from build123d import *

# Parameters (mm, degrees)
SKETCH067_R             = 1.875
PAD035_DEPTH            = 4.75
SKETCH068_R             = 3
POCKET007018_DEPTH      = 3.75
POCKET007019_DEPTH      = 3.5
FILLET001_R             = 3
BODY008_PLACEMENT_ANGLE = 180


with BuildPart() as part:
    # Sketch067 → Pad035 (new body)
    with BuildSketch(Plane.XY.offset(-4)):
        with BuildLine():
            Line((17, -30.839247), (30.583921, -30.839247))
            Line((30.583921, -30.839247), (30.583921, -40.999999))
            ThreePointArc((30.583921, -40.999999), (36.500001, -45.999999), (42.416081, -40.999999))
            Line((42.416081, -30.839247), (42.416081, -40.999999))
            Line((42.416081, -30.839247), (55.233103, -30.839247))
            Line((55.233103, -30.839247), (83.336753, 5.788599))
            Line((83.336753, 5.788599), (75.403023, 11.875956))
            Line((75.403023, 11.875956), (48.766897, -22.839247))
            Line((48.766897, -22.839247), (17, -22.839247))
            Line((17, -22.839247), (17, -30.839247))
        make_face()
        with Locations((21, -26.839247)):
            Circle(SKETCH067_R, mode=Mode.SUBTRACT)
        with Locations((52, -26.839247)):
            Circle(SKETCH067_R, mode=Mode.SUBTRACT)
        with BuildLine():
            ThreePointArc((38.875001, -34.999999), (36.500001, -32.624999), (34.125001, -34.999999))
            Line((34.125001, -34.999999), (34.125001, -40.999999))
            ThreePointArc((34.125001, -40.999999), (36.500001, -43.374999), (38.875001, -40.999999))
            Line((38.875001, -34.999999), (38.875001, -40.999999))
        make_face(mode=Mode.SUBTRACT)
        with BuildLine():
            ThreePointArc((77.601735, 2.626292), (77.163221, 5.9563), (73.833213, 5.517786))
            Line((73.833213, 5.517786), (70.789534, 1.550921))
            ThreePointArc((70.789534, 1.550921), (71.228048, -1.779087), (74.558056, -1.340574))
            Line((77.601735, 2.626292), (74.558056, -1.340574))
        make_face(mode=Mode.SUBTRACT)
    extrude(amount=PAD035_DEPTH)

    # Sketch068 (on ShapeBinder) → Pocket007018 (cut)
    with BuildSketch(Plane(origin=(-1.5, -35, 0.75), x_dir=(0, 1, 0), z_dir=(0, 0, -1))):
        with Locations((8.353044, 53.594845)):
            Circle(SKETCH068_R)
        with Locations((8.160753, 22.5)):
            Circle(SKETCH068_R)
    extrude(amount=POCKET007018_DEPTH, mode=Mode.SUBTRACT)

    # Sketch069 → Pocket007019 (cut)
    with BuildSketch(Plane.XY.offset(-4)):
        Polygon((40.125001, -37.092894), (40.125001, -32.907104), (36.500001, -30.814209), (32.875001, -32.907104), (32.875001, -37.092894), (32.875001, -38.907104), (32.875001, -43.092894), (36.500001, -45.185788), (40.125001, -43.092894), (40.125001, -38.907104), align=None)
        Polygon((77.319431, 0.204926), (79.867471, 3.525818), (78.265513, 7.392932), (74.115516, 7.939152), (71.567477, 4.61826), (71.071837, 3.972287), (68.523798, 0.651395), (70.125755, -3.215719), (74.275752, -3.76194), (76.823792, -0.441047), align=None)
    extrude(amount=POCKET007019_DEPTH, mode=Mode.SUBTRACT)

    # Fillet001
    fillet001_edges = [part.edges().sort_by_distance(p)[0] for p in [
        (42.416081, -30.839247, -1.625),
        (55.233103, -30.839247, -1.625),
        (83.336753, 5.788599, -1.625),
        (75.403023, 11.875956, -1.625),
        (48.766897, -22.839247, -1.625),
        (17, -22.839247, -1.625),
        (17, -30.839247, -1.625),
        (30.583921, -30.839247, -1.625),
    ]]
    fillet(fillet001_edges, radius=FILLET001_R)


with BuildPart() as part_1:
    # Body008 placement: moved
    add(part.part.rotate(Axis((0, 0, 0), (1, 0, 0)), BODY008_PLACEMENT_ANGLE))


solid = part_1.part
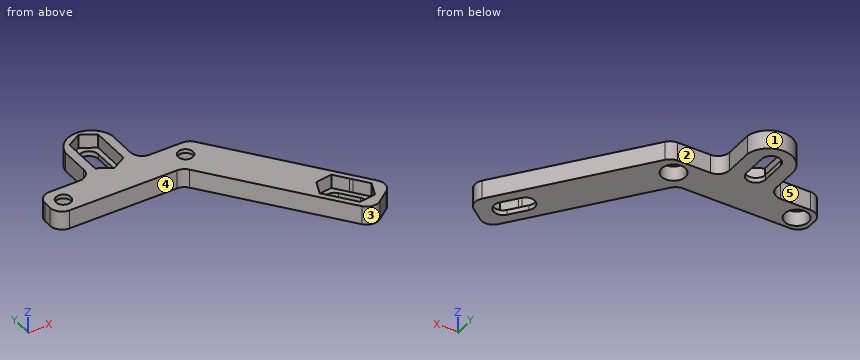
For this review, take the finished solid that the model builds, in its own axes (mm). Face numbers are marked on the shaded views. A direction names the side the tool comes from. Round coordinates to 2 decimals unless told otherwise and drop trailing zeros. Loops run counter-clockwise (first coordinate to the right, second up) from the corner with the lowest first, then second, coordinate; pieces in that order, holes last. Notation, with made-up numbers: (-11.75, 64.25) - (17.25, 64.25) arc R29 cw to (17.25, 87.25) - close; hole circle Ø6 at (11.25, 78). An arc over 180 degrees is marked (long way). Put each result on its own line as item: value. Start each with the question number.
1. Consider section C-C on z = 1.45. State how many separate pieces and enclosed holes the cut face has, plus the area to 3 significant figures.
2. For the marked faces 1, 2, 3, 4 and 5, list the 3-axis set-ups (+Z, -Z, +X, -X, +Y, -Y) from which the entire face can be reached by the end or side of a thin tool; tool diameter is ignored.
3. Consider section A-A on x = 21. State the section outline as (y, z) points.
4. For probe 1 along X at (y, z) = (38, 3.2) (3 decimals); probe 2 along Y at (x, z) = (21, 3.75); probe 3 along Y at (x, z) = (50.5, 1.85), list the stretches that pass through material, from the lowest coordinate up. Write a range as [from, to].
5. Insertion check: P1, Ø9, axis at x = 74, y = -4.5, coming from the +Z side; P2, Ø2, axis at x = 62.5, z = 2, coming from the +Y side; P3, Ø1.4, axis at y = 39, z = 2.5, coming from the -X side; P4, Ø1.8, axis at x = 53, y = 28, coming from the -Z side. Each pin has a flat end and moves straight along its axis. Give the tip position at first contact, or say it passes through.
6. Consider section B-B on x = 67. State the section outline as (y, z) points.
7. Consider section D-D on x = 48. State the section outline as (y, z) points, plus the area to 3 significant figures.
Result sheet:
1. separate pieces: 1
1. enclosed holes: 4
1. area: 663 mm^2
2. face 1: +Z, -Z, +Y
2. face 2: +Z, -Z, +X, +Y
2. face 3: +Z, -Z, -Y
2. face 4: +Z, -Z, -X, -Y
2. face 5: +Z, -Z, -X, +Y
3. outline: (22.84, -0.75) - (23.84, -0.75) - (23.84, 3) - (24.96, 3) - (24.96, 4) - (22.84, 4) - close; (28.71, 3) - (29.84, 3) - (29.84, -0.75) - (30.84, -0.75) - (30.84, 4) - (28.71, 4) - close
4. probe 1: [30.584, 32.875], [40.125, 42.416]
4. probe 2: [22.84, 24.96], [28.71, 30.84]
4. probe 3: [20.58, 24.11], [29.19, 30.84]
5. P1: z = 4
5. P2: y = 22.67
5. P3: x = 30.58
5. P4: z = 3
6. outline: (-0.92, -0.75) - (15.5, -0.75) - (15.5, 4) - (-0.92, 4) - close
7. outline: (22.75, -0.75) - (30.84, -0.75) - (30.84, 4) - (22.75, 4) - close
7. area: 38.4 mm^2
